Can you work these out from the model? Positions are in its coordinate system, mm. A direction names the side the tool comes from. Coordinates: 2 decimals unless noted, no trailing zeros. Loops run counter-clockwise (first coordinate to the right, second up) from the corner with the lowest first, then second, coordinate; pieces in that order, holes last.
```python
from build123d import *

# Parameters (mm, degrees)
SKETCH1_R           = 31.5
BOSS_EXTRUDE1_DEPTH = 2
SKETCH2_R           = 1
SKETCH2_R_2         = 1.2
CUT_EXTRUDE2_DEPTH  = 3
SKETCH5_R           = 1
BOSS_EXTRUDE3_DEPTH = 1
BOSS_EXTRUDE2_DEPTH = 30
CUT_EXTRUDE3_DEPTH  = 32.5


with BuildPart() as part:
    # Sketch1 → Boss-Extrude1 (new body)
    with BuildSketch(Plane.XY):
        Circle(SKETCH1_R)
        with BuildLine():
            Line((-12.757350822, -21.5), (12.757350822, -21.5))
            ThreePointArc((12.757350822, -21.5), (13.509438116, -21.035567066), (14.244636813, -20.544836871))
            ThreePointArc((14.244636813, -20.544836871), (15.464466094, -15.464466094), (20.544836871, -14.244636813))
            ThreePointArc((20.544836871, -14.244636813), (25, 0), (20.544836871, 14.244636813))
            ThreePointArc((20.544836871, 14.244636813), (15.464466094, 15.464466094), (14.244636813, 20.544836871))
            ThreePointArc((14.244636813, 20.544836871), (11.482464544, 22.207048611), (8.529361055, 23.5))
            Line((8.529361055, 23.5), (-8.529361055, 23.5))
            ThreePointArc((-8.529361055, 23.5), (-11.482464544, 22.207048611), (-14.244636813, 20.544836871))
            ThreePointArc((-14.244636813, 20.544836871), (-15.464466094, 15.464466094), (-20.544836871, 14.244636813))
            ThreePointArc((-20.544836871, 14.244636813), (-25, 0), (-20.544836871, -14.244636813))
            ThreePointArc((-20.544836871, -14.244636813), (-15.464466094, -15.464466094), (-14.244636813, -20.544836871))
            ThreePointArc((-14.244636813, -20.544836871), (-13.509438116, -21.035567066), (-12.757350822, -21.5))
        make_face(mode=Mode.SUBTRACT)
    extrude(amount=BOSS_EXTRUDE1_DEPTH)

    # Sketch2 → Cut-Extrude2 (cut, through all)
    with BuildSketch(Plane.XY):
        with Locations((-19, 19)):
            Circle(SKETCH2_R)
        with Locations((-16.8, 16.8)):
            Circle(SKETCH2_R)
        with Locations((19, 19)):
            Circle(SKETCH2_R)
        with Locations((16.8, 16.8)):
            Circle(SKETCH2_R)
        with Locations((-19, -19)):
            Circle(SKETCH2_R)
        with Locations((-16.8, -16.8)):
            Circle(SKETCH2_R)
        with Locations((19, -19)):
            Circle(SKETCH2_R)
        with Locations((16.8, -16.8)):
            Circle(SKETCH2_R)
        with Locations((-28, 0)):
            Circle(SKETCH2_R_2)
        with Locations((28, 0)):
            Circle(SKETCH2_R_2)
        with Locations((0, 28)):
            Circle(SKETCH2_R_2)
        with Locations((0, -28)):
            Circle(SKETCH2_R_2)
    extrude(amount=CUT_EXTRUDE2_DEPTH, mode=Mode.SUBTRACT)

    # Sketch5 → Boss-Extrude3 (add)
    with BuildSketch(Plane(origin=(0, 0, 0), x_dir=(-1, 0, 0), z_dir=(0, 0, -1))):
        with BuildLine():
            Line((-17.664466094, 20.335533906), (-15.464466094, 18.135533906))
            ThreePointArc((-15.464466094, 18.135533906), (-15.464466094, 15.464466094), (-18.135533906, 15.464466094))
            Line((-18.135533906, 15.464466094), (-20.335533906, 17.664466094))
            ThreePointArc((-20.335533906, 17.664466094), (-20.335533906, 20.335533906), (-17.664466094, 20.335533906))
        make_face()
        with Locations((-19, 19)):
            Circle(SKETCH5_R, mode=Mode.SUBTRACT)
        with Locations((-16.8, 16.8)):
            Circle(SKETCH5_R, mode=Mode.SUBTRACT)
        with BuildLine():
            Line((20.335533906, 17.664466094), (18.135533906, 15.464466094))
            ThreePointArc((18.135533906, 15.464466094), (15.464466094, 15.464466094), (15.464466094, 18.135533906))
            Line((15.464466094, 18.135533906), (17.664466094, 20.335533906))
            ThreePointArc((17.664466094, 20.335533906), (20.335533906, 20.335533906), (20.335533906, 17.664466094))
        make_face()
        with Locations((16.8, 16.8)):
            Circle(SKETCH5_R, mode=Mode.SUBTRACT)
        with Locations((19, 19)):
            Circle(SKETCH5_R, mode=Mode.SUBTRACT)
        with BuildLine():
            Line((17.664466094, -20.335533906), (15.464466094, -18.135533906))
            ThreePointArc((15.464466094, -18.135533906), (15.464466094, -15.464466094), (18.135533906, -15.464466094))
            Line((18.135533906, -15.464466094), (20.335533906, -17.664466094))
            ThreePointArc((20.335533906, -17.664466094), (20.335533906, -20.335533906), (17.664466094, -20.335533906))
        make_face()
        with Locations((16.8, -16.8)):
            Circle(SKETCH5_R, mode=Mode.SUBTRACT)
        with Locations((19, -19)):
            Circle(SKETCH5_R, mode=Mode.SUBTRACT)
        with BuildLine():
            Line((-20.335533906, -17.664466094), (-18.135533906, -15.464466094))
            ThreePointArc((-18.135533906, -15.464466094), (-15.464466094, -15.464466094), (-15.464466094, -18.135533906))
            Line((-15.464466094, -18.135533906), (-17.664466094, -20.335533906))
            ThreePointArc((-17.664466094, -20.335533906), (-20.335533906, -20.335533906), (-20.335533906, -17.664466094))
        make_face()
        with Locations((-16.8, -16.8)):
            Circle(SKETCH5_R, mode=Mode.SUBTRACT)
        with Locations((-19, -19)):
            Circle(SKETCH5_R, mode=Mode.SUBTRACT)
    extrude(amount=BOSS_EXTRUDE3_DEPTH)

    # Sketch3 → Boss-Extrude2 (add)
    with BuildSketch(Plane.XY):
        with BuildLine():
            Line((-10.924320544, 23.5), (10.924320544, 23.5))
            ThreePointArc((10.924320544, 23.5), (14.757350822, 24.3), (10.924320544, 25.1))
            Line((10.924320544, 25.1), (-10.924320544, 25.1))
            ThreePointArc((-10.924320544, 25.1), (-14.757350822, 24.3), (-10.924320544, 23.5))
        make_face()
        with BuildLine():
            Line((-12.757350822, -21.5), (12.757350822, -21.5))
            ThreePointArc((12.757350822, -21.5), (14.171564385, -24.914213562), (10.757350822, -23.5))
            Line((10.757350822, -23.5), (-10.757350822, -23.5))
            ThreePointArc((-10.757350822, -23.5), (-14.171564385, -24.914213562), (-12.757350822, -21.5))
        make_face()
    extrude(amount=BOSS_EXTRUDE2_DEPTH)

    # Sketch4 → Cut-Extrude3 (cut, through all)
    with BuildSketch(Plane(origin=(0, 0, 0), x_dir=(1, 0, 0), z_dir=(0, 1, 0))):
        Polygon((-11, -30), (-11, -24), (-8, -24), (-3, -4), (3, -4), (8, -24), (11, -24), (11, -30), align=None)
    extrude(amount=CUT_EXTRUDE3_DEPTH, mode=Mode.SUBTRACT)


solid = part.part
```
Item 1: I'm going to push flat-ended pins straight in: P1, Ø11, axis at x = -0.5, z = 10, coming from the -Y side; P2, Ø3, axis at x = 19, y = 19, coming from the +Z side; P3, Ø2.5, axis at x = -16.8, y = -16.8, coming from the -Z side; P4, Ø1, axis at x = -11.5, z = 17.5, coming from the -Y side. Where does each tip first touch, or does it pass through?
Results are:
P1: stops at y = -23.5
P2: stops at z = 2
P3: stops at z = -1
P4: stops at y = -25.35
Item 2: Suppose I cut it at A-A, the plane z = 11. Please give me the cut outline in (x, y).
Results are:
outline: (-12.76, -21.5) arc R2 ccw (long way) to (-10.76, -23.5) - (10.76, -23.5) arc R2 ccw (long way) to (12.76, -21.5) - close; (-10.92, 23.5) - (-4.75, 23.5) - (-4.75, 25.1) - (-10.92, 25.1) arc R2 ccw (long way) to start; (4.75, 23.5) - (10.92, 23.5) arc R2 ccw (long way) to (10.92, 25.1) - (4.75, 25.1) - close
Item 3: On a 3-axis mill with a long thin cutter (end or side, diameter ignored), from which of +Z, -Z, +X, -X, +Y, -Y can I reach the whole of each face in a straight line? I mean faces 1 (the face through (-20.31, 20.36, -0.49)), 2 (the face through (-25, 0, 1)), 3 (the face through (5.465, 24.289, 13.86)), 4 (the face through (-14.124, -24.96, 15.804)). Say none if no direction works.
Results are:
face 1: -Z
face 2: +Z, -Z
face 3: +Z, +Y
face 4: +Z
Item 4: I need wall thicknesses on line 1 along Y through (x, z) = (0, 1.15); line 2 along Y through (x, z) = (16, 1); line 3 along X through (y, z) = (19, 0.45). Which ranges of each line are inside material? Lowest first, please.
Results are:
line 1: y = -31.5 to -29.2, -26.8 to -21.5, 23.5 to 26.8, 29.2 to 31.5
line 2: y = -27.13 to -17.4, -16.2 to -15, 15 to 16.2, 17.4 to 27.13
line 3: x = -25.12 to -20, -18 to -14, 14 to 18, 20 to 25.12
Item 5: Suppose I cut it at D-D, the plane y = 12. Please give me the cut outline in (x, z).
Results are:
outline: (-29.12, 0) - (-21.93, 0) - (-21.93, 2) - (-29.12, 2) - close; (21.93, 0) - (29.12, 0) - (29.12, 2) - (21.93, 2) - close
Item 6: Suppose I cut it at C-C, the plane y = 0. Please give me the cut outline in (x, z).
Results are:
outline: (-31.5, 0) - (-29.2, 0) - (-29.2, 2) - (-31.5, 2) - close; (-26.8, 0) - (-25, 0) - (-25, 2) - (-26.8, 2) - close; (25, 0) - (26.8, 0) - (26.8, 2) - (25, 2) - close; (29.2, 0) - (31.5, 0) - (31.5, 2) - (29.2, 2) - close
Item 7: Suppose I cut it at B-B, the plane x = 0. Please give me the cut outline in (y, z), plus the area to 3 significant figures.
Results are:
outline: (-31.5, 0) - (-29.2, 0) - (-29.2, 2) - (-31.5, 2) - close; (-26.8, 0) - (-21.5, 0) - (-21.5, 30) - (-23.5, 30) - (-23.5, 2) - (-26.8, 2) - close; (23.5, 0) - (26.8, 0) - (26.8, 2) - (25.1, 2) - (25.1, 4) - (23.5, 4) - close; (29.2, 0) - (31.5, 0) - (31.5, 2) - (29.2, 2) - close
area: 85.6 mm2
Item 8: We'd pull the mould along Y, two halves only. Please class faces 5 (the face through (-16.55, 19.22, -0.49)), 6 (the face through (11.5, 22.2, 1)), 7 (the face through (-18, -18, -1)): +Y half, -Y half, draft (parallel to the pull), parting line (faces both ways), or undercut.
Results are:
face 5: +Y half
face 6: undercut
face 7: draft
